The drawing under review shows one solid part. Ordinate dimensions are in mm from its lowest x, y, z. Coordinates: 2 decimals unless noted, no trailing zeros. Loops run counter-clockwise (first coordinate to the right, second up) from the corner with the lowest first, then second, coordinate; pieces in that order, holes last. Notation, with made-up numbers: M -16.5,-6.5 L -2.5,-6.5 A9 cw -2.5,-2.5 Z; hole C -21.5,37.25 d1. An arc over 180 degrees is marked long. Return JSON: item names as keys, results as strings.
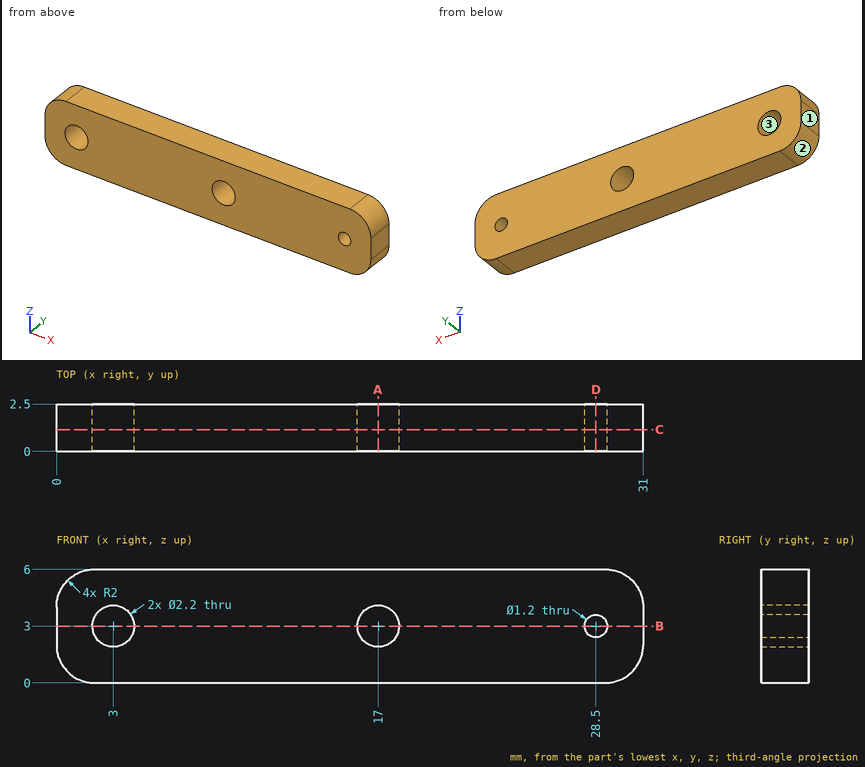
1. Add section D-D on x = 28.5. Give the boundary of the cut face in (y, z).
Check values:
{"outline": "M 0,0 L 2.5,0 L 2.5,2.4 L 0,2.4 Z; M 0,3.6 L 2.5,3.6 L 2.5,6 L 0,6 Z"}
2. Insertion check: pin 1 Ø2.5 at (x, z) = (17, 3) entering from -Y. The pin has a flat end and moves straight along its axis. Give the tip position at first contact, or say it passes through.
Check values:
{"pin 1": "y = 0"}
3. Add section B-B on z = 3. Give the boundary of the cut face in (x, y).
Check values:
{"outline": "M 0,0 L 1.9,0 L 1.9,2.5 L 0,2.5 Z; M 4.1,0 L 15.9,0 L 15.9,2.5 L 4.1,2.5 Z; M 18.1,0 L 27.9,0 L 27.9,2.5 L 18.1,2.5 Z; M 29.1,0 L 31,0 L 31,2.5 L 29.1,2.5 Z"}
4. Add section C-C on y = 1.15. Give the boundary of the cut face in (x, z), plus the area to 3 significant figures.
Check values:
{"outline": "M 0,2 A2 ccw 2,0 L 29,0 A2 ccw 31,2 L 31,4 A2 ccw 29,6 L 2,6 A2 ccw 0,4 Z; hole C 3,3 d2.2; hole C 17,3 d2.2; hole C 28.5,3 d1.2", "area": "174 mm²"}
5. The part is to be moulded in two halves that separate along Z. For the marked faces 1, 2 and 3, say which applies: released by +Z, released by -Z, zero draft, split by the parting line, or undercut.
Check values:
{"face 1": "zero draft", "face 2": "released by -Z", "face 3": "undercut"}
6. To check wall thickness, follow line 1 (X direction, y = 0.95, z = 3); line 2 (X direction, y = 1.8, z = 3.5); line 3 (X direction, y = 1.2, z = 3.75). State the ranges of each line that lie inside material, in increasing order.
Check values:
{"line 1": "0 to 1.9, 4.1 to 15.9, 18.1 to 27.9, 29.1 to 31", "line 2": "0 to 2.02, 3.98 to 16.02, 17.98 to 28.17, 28.83 to 31", "line 3": "0 to 2.2, 3.8 to 16.2, 17.8 to 31"}
7. Add section A-A on x = 17. Give the boundary of the cut face in (y, z).
Check values:
{"outline": "M 0,0 L 2.5,0 L 2.5,1.9 L 0,1.9 Z; M 0,4.1 L 2.5,4.1 L 2.5,6 L 0,6 Z"}
